The drawing under review shows one solid part. Ordinate dimensions are in mm from its lowest x, y, z. A direction names the side the tool comes from. Give positions to 0.01 mm unless a question says otherwise; leave off trailing zeros. Order: outer loops, then holes, each group sorted by start corner. A loop starts at its lowest first (then second) coordinate and runs counter-clockwise, first axis right, second up. Notation, with made-up numbers: (58.25, 74.5) -> (96.25, 74.5) arc R21 ccw to (96.25, 107.5) -> close; hole circle Ø4 at (50.25, -35.5). An arc over 180 degrees is marked (long way). Use a Markdown table: item, result. Add a question column.
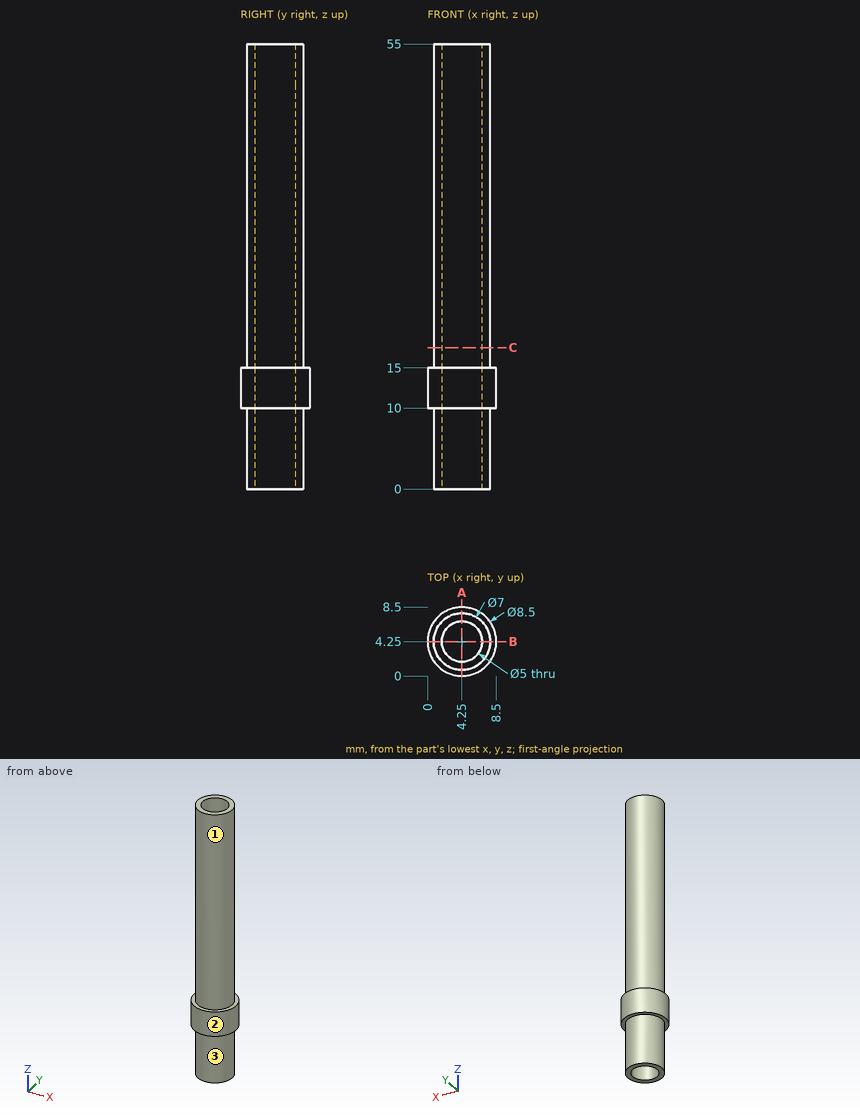
1) Add section A-A (x = 4.25). Give the boundary of the cut face in (y, z), then the cut area to 4 significant figures.
2) Insertion check: pin 1 (3 mm diameter, centred on x = 4.25, y = 4.25, fed in from -Z); pin 2 (1 mm diameter, centred on x = 7, z = 42.5, fed in from +Y); pin 3 (3 mm diameter, centred on y = 2, z = 47, fed in from -X); pin 4 (5 mm diameter, centred on x = 6, z = 22, fed in from -Y). Each pin has a flat end and moves straight along its axis. Give the tip position at first contact, or say it passes through.
3) Machinability: for the marked faces 1, 2 and 3, which of the approach directions +Z, -Z, +X, -X, +Y, -Y give a long, thin tool a straight path to every point of the face, cutting with its end or side? Answer none if there is none.
4) For L1, parallel to Y at x = 4.25, z = 2.5; L2, parallel to Z at x = 6.75, y = 1.25, list the stretches that pass through material, from the lowest coordinate up. Write a range as [from, to].
5) Add section C-C (z = 17.5). Give the boundary of the cut face in (x, y).
Worked answers:
| question | item | result |
|---|---|---|
| 1 | outline | (0, 10) -> (0.75, 10) -> (0.75, 0) -> (1.75, 0) -> (1.75, 55) -> (0.75, 55) -> (0.75, 15) -> (0, 15) -> close; (6.75, 0) -> (7.75, 0) -> (7.75, 10) -> (8.5, 10) -> (8.5, 15) -> (7.75, 15) -> (7.75, 55) -> (6.75, 55) -> close |
| 1 | area | 117.5 mm^2 |
| 2 | pin 1 | through |
| 2 | pin 2 | y = 6.93 |
| 2 | pin 3 | x = 0.83 |
| 2 | pin 4 | y = 0.75 |
| 3 | face 1 | +Z |
| 3 | face 2 | +Z, -Z |
| 3 | face 3 | -Z |
| 4 | L1 | [0.75, 1.75], [6.75, 7.75] |
| 4 | L2 | [10, 15] |
| 5 | outline | circle Ø7 at (4.25, 4.25); hole circle Ø5 at (4.25, 4.25) |
